Part model, mm, in its own coordinate system. A direction names the side the tool comes from. Round coordinates to 2 decimals unless told otherwise and drop trailing zeros. Write each loop counter-clockwise with the first axis right and the second up, starting at its lowest first coordinate (ties: lowest second). Pieces come first, ordered by that corner, then holes. Notation, with made-up numbers: M 68,-10.5 L 92,-10.5 A4 cw 92,-5.5 Z; hole C 50.5,28 d10. An arc over 180 degrees is marked long. Use a Markdown table: item, result. Add a question column.
1) Slice it at B-B on y = -5.5. Write the cut outline in (x, z), plus the area to 3 significant figures.
2) Wall check: probe 1 along Z at (x, y) = (8.5, 1.25); probe 2 along X at (y, z) = (-5.75, 12); probe 3 along Y at (x, z) = (-14, 26). Give the ranges that are in metal, low to high.
3) Which spindle directions (+Z, -Z, +X, -X, +Y, -Y) get a long thin tool onto all of the face, cutting with end or side? Do faces 1 (the face through (13.75, -6, 16)), 2 (the face through (14, 2.784, 17)), 3 (the face through (11.9, 5, 16)). Say none if no direction does.
4) Slice it at C-C on x = -10. Write the cut outline in (y, z).
5) Slice it at A-A on z = 24.5. Write the cut outline in (x, y), plus the area to 3 significant figures.
6) Two-plate mould, pull along Y, no slides. Class faces 4 (the face through (16.75, -1, 17)), 5 (the face through (-16.18, 7.18, 17.24)), 6 (the face through (15.879, -1.433, 34.073)), 7 (the face through (-14, 2.784, 17)): released by +Y, released by -Y, zero draft, split by the parting line, or undercut.
7) Drop flat-ended pins along their axis: P1, Ø6.5, axis at x = 1, y = -3.5, coming from the +Z side; P2, Ø11.5, axis at x = 1, z = 27.5, coming from the +Y side; P3, Ø1.5, axis at x = 2.5, y = 0, coming from the +Z side; P4, Ø13, axis at x = -3, z = 16.5, coming from the -Y side. Give the stop position or say it passes through.
```python
from build123d import *

# Parameters (mm, degrees)
BOSS_EXTRU_1_DEPTH      = 33
ESQUISSE2_W             = 4
ESQUISSE2_H             = 2.5
ENL_V_MAT_EXTRU_1_DEPTH = 48.736346803
ESQUISSE3_W             = 4
ESQUISSE3_H             = 2.5
ENL_V_MAT_EXTRU_2_DEPTH = 48.736346803
ESQUISSE4_W             = 33.5
ESQUISSE4_H             = 7.783625731
BOSS_EXTRU_2_DEPTH      = 3
CHANFREIN1_SIZE         = 3
CONG_3_START            = -18
CONG_3_DEPTH            = 36
CONG_2_R                = 2


with BuildPart() as part:
    # Esquisse1 → Boss.-Extru.1 (new body)
    with BuildSketch(Plane.XY):
        Polygon((-11.9, 2.783625731), (11.9, 2.783625731), (11.9, 7.783625731), (16.75, 7.783625731), (16.75, -8.216374269), (13.75, -8.216374269), (13.75, -3.216374269), (-13.75, -3.216374269), (-13.75, -8.216374269), (-16.75, -8.216374269), (-16.75, 7.783625731), (-11.9, 7.783625731), align=None)
    extrude(amount=BOSS_EXTRU_1_DEPTH)

    # Esquisse2 → Enlèv. mat.-Extru.1 (cut, through all)
    with BuildSketch(Plane(origin=(16.75, 0, 0), x_dir=(0, 0, -1), z_dir=(1, 0, 0))):
        with Locations((-24.5, -1.966374269)):
            Rectangle(ESQUISSE2_W, ESQUISSE2_H)
        with Locations((-8.5, -1.966374269)):
            Rectangle(ESQUISSE2_W, ESQUISSE2_H)
    extrude(amount=-ENL_V_MAT_EXTRU_1_DEPTH, mode=Mode.SUBTRACT)

    # Esquisse3 → Enlèv. mat.-Extru.2 (cut, through all)
    with BuildSketch(Plane(origin=(16.75, 0, 0), x_dir=(0, 0, -1), z_dir=(1, 0, 0))):
        with Locations((-16.5, 1.533625731)):
            Rectangle(ESQUISSE3_W, ESQUISSE3_H)
    extrude(amount=-ENL_V_MAT_EXTRU_2_DEPTH, mode=Mode.SUBTRACT)

    # Esquisse4 → Boss.-Extru.2 (add)
    with BuildSketch(Plane.XY.offset(33)):
        with Locations((0, 3.891812866)):
            Rectangle(ESQUISSE4_W, ESQUISSE4_H)
    extrude(amount=BOSS_EXTRU_2_DEPTH)

    # Chanfrein1
    chanfrein1_edges = [part.edges().sort_by_distance(p)[0] for p in [
        (0, 0, 33),
    ]]
    chamfer(chanfrein1_edges, length=CHANFREIN1_SIZE - 0.0001)  # a hair under: the kernel refuses the full size

    # Congé3: read off the stored shape, not the designer's step
    # Congé3 outline → Congé3 (cut)
    with BuildSketch(Plane.YZ.offset(CONG_3_START)):
        with BuildLine():
            Line((0, 36), (-0.878679656, 35.121320344))
            ThreePointArc((-0.878679656, 35.121320344), (0.09459039, 35.771638598), (1.242640687, 36))
            Line((1.242640687, 36), (0, 36))
        make_face()
    extrude(amount=CONG_3_DEPTH, mode=Mode.SUBTRACT)

    # Congé2
    cong_2_edges = [part.edges().sort_by_distance(p)[0] for p in [
        (0, 7.783625731, 36),
        (-16.75, -1.931982494, 34.067917506),
        (16.75, 4.513133209, 36),
        (16.75, -1.931982494, 34.067917506),
        (16.75, 0.104112039, 35.77556346),
        (-16.75, 0.104112039, 35.77556346),
        (16.75, 7.783625731, 18),
        (-16.75, 7.783625731, 18),
        (-16.75, 4.513133209, 36),
    ]]
    fillet(cong_2_edges, radius=CONG_2_R)


solid = part.part
```
Entries:
| question | item | result |
|---|---|---|
| 1 | outline | M -16.75,0 L -13.75,0 L -13.75,33 L -16.75,33 Z; M 13.75,0 L 16.75,0 L 16.75,33 L 13.75,33 Z |
| 1 | area | 198 mm^2 |
| 2 | probe 1 | z = 0 to 14.5, 18.5 to 36 |
| 2 | probe 2 | x = -16.75 to -13.75, 13.75 to 16.75 |
| 2 | probe 3 | y = -8.22 to -3.22, -0.72 to 7.78 |
| 3 | face 1 | +Z, -Z, -Y |
| 3 | face 2 | +X, -X |
| 3 | face 3 | -Z, +Y |
| 4 | outline | M -3.22,0 L 2.78,0 L 2.78,14.5 L 0.28,14.5 L 0.28,18.5 L 2.78,18.5 L 2.78,33 L 7.78,33 L 7.78,34 A2 ccw 5.78,36 L 1.24,36 A3 ccw -0.86,35.14 L -3,33 L -3.22,33 L -3.22,26.5 L -0.72,26.5 L -0.72,22.5 L -3.22,22.5 L -3.22,10.5 L -0.72,10.5 L -0.72,6.5 L -3.22,6.5 Z |
| 5 | outline | M -16.75,-8.22 L -13.75,-8.22 L -13.75,-3.22 L -16.75,-3.22 Z; M -16.75,-0.72 L 16.75,-0.72 L 16.75,5.78 A2 ccw 14.75,7.78 L 11.9,7.78 L 11.9,2.78 L -11.9,2.78 L -11.9,7.78 L -14.75,7.78 A2 ccw -16.75,5.78 Z; M 13.75,-8.22 L 16.75,-8.22 L 16.75,-3.22 L 13.75,-3.22 Z |
| 5 | area | 194 mm^2 |
| 6 | face 4 | zero draft |
| 6 | face 5 | released by +Y |
| 6 | face 6 | released by -Y |
| 6 | face 7 | undercut |
| 7 | P1 | stops at z = 35.6 |
| 7 | P2 | stops at y = 7.78 |
| 7 | P3 | stops at z = 35.96 |
| 7 | P4 | stops at y = -3.22 |
